Geometry check sheet. Reference: the model listing, model coordinates, mm. Coordinates: 2 decimals unless noted, no trailing zeros. Answer in a Markdown table with one row per item. Add a question column.
1. Cross-section at A-A on y = 5.5. Give the number of separate pieces and of enclosed holes in the cut face, and give its area (3 significant figures).
2. Depth check by flat-ended pin: P1, Ø7, axis at x = 6, z = 362.5, coming from the -Y side; P2, Ø4, axis at x = 6, z = 212.5, coming from the +Y side; P3, Ø3, axis at x = 6, z = 262.5, coming from the +Y side. Enter the tip coordinate at first touch or a pass-through.
3. Scan lines: L1, parallel to X at y = 5.65, z = 287.5; L2, parallel to X at y = 2.3, z = 287.5. Record each from-to range of solid material in increasing order. Write a range as from..to.
```python
from build123d import *

# Parameters (mm, degrees)
SKETCH1_W           = 12
SKETCH1_H           = 8
BOSS_EXTRUDE1_DEPTH = 400
SKETCH2_R           = 3
CUT_EXTRUDE1_DEPTH  = 4.5
SKETCH4_R           = 1.75
CUT_EXTRUDE2_DEPTH  = 401.259915555
LPATTERN2_COUNT     = 16
LPATTERN2_PITCH     = 25


with BuildPart() as part:
    # Sketch1 → Boss-Extrude1 (new body)
    with BuildSketch(Plane.XY):
        with Locations((6, 4)):
            Rectangle(SKETCH1_W, SKETCH1_H)
    extrude(amount=BOSS_EXTRUDE1_DEPTH)

    # Sketch2 → Cut-Extrude1 (cut)
    with BuildSketch(Plane(origin=(0, 8, 0), x_dir=(1, 0, 0), z_dir=(0, 1, 0))):
        with Locations(Location((6, -12.5, 0), (0, 0, 270))):
            Circle(SKETCH2_R)
    cut_extrude1 = extrude(amount=-CUT_EXTRUDE1_DEPTH, mode=Mode.SUBTRACT)

    # Sketch4 → Cut-Extrude2 (cut, through all)
    with BuildSketch(Plane.XZ):
        with Locations(Location((6, 12.5, 0), (0, 0, 270))):
            Circle(SKETCH4_R)
    cut_extrude2 = extrude(amount=-CUT_EXTRUDE2_DEPTH, mode=Mode.SUBTRACT)

    # LPattern2: Cut-Extrude1, Cut-Extrude2 ×16
    with Locations(*[(0, 0, i * LPATTERN2_PITCH) for i in range(1, LPATTERN2_COUNT)]):
        add(cut_extrude1, mode=Mode.SUBTRACT)
        add(cut_extrude2, mode=Mode.SUBTRACT)


solid = part.part
```
Results found:
| question | item | result |
|---|---|---|
| 1 | separate pieces | 1 |
| 1 | enclosed holes | 16 |
| 1 | area | 4,350 mm^2 |
| 2 | P1 | stops at y = 0 |
| 2 | P2 | stops at y = 3.5 |
| 2 | P3 | passes through |
| 3 | L1 | x = 0..3, 9..12 |
| 3 | L2 | x = 0..4.25, 7.75..12 |
